Autodesk Inventor part; units mm, degrees
ref_plane "YZ Plane" through (0, 0, 0) normal (1, 0, 0) x (0, 1, 0)
ref_plane "XZ Plane" through (0, 0, 0) normal (0, 1, 0) x (-1, 0, 0)
ref_plane "XY Plane" through (0, 0, 0) normal (0, 0, 1) x (1, 0, 0)
sketch "Szkic3" plane through (0, 0, 0) normal (0, 1, 0) x (-1, 0, 0)
  line L0 (0, 0) -> (10, 0)
  line L1 (10, 0) -> (10, -50)
  line L2 (10, -50) -> (0, -50)
  line L3 (0, -50) -> (0, 0)
  circle A0 centre (5, -5) radius 2.5
  arc A1 (10, -2.5) -> (0, -2.5) centre (5, -6.25) ccw
  line L4 (8, -50) -> (2, -50)
  line L5 (2, -50) -> (2, -10)
  line L6 (2, -10) -> (8, -10)
  line L7 (8, -10) -> (8, -50)
  line L8 (2, -10) -> (8, -16)
  line L9 (2, -10) -> (10.4853, -10) construction
  line L10 (8, -16) -> (8, -18)
  line L11 (8, -18) -> (2, -12)
  line L12 (2, -10) -> (2, -12)
  line L13 (8, -18) -> (8, -22)
  line L14 (2, -16) -> (8, -22)
  line L15 (8, -24) -> (2, -18)
  line L16 (8, -16) -> (8, -14)
  line L17 (8, -24) -> (8, -26)
  line L18 (2, -20) -> (8, -26)
  line L19 (8, -28) -> (2, -22)
  line L20 (8, -28) -> (8, -32)
  line L21 (2, -26) -> (8, -32)
  line L22 (8, -34) -> (2, -28)
  line L23 (8, -34) -> (8, -36)
  line L24 (2, -26) -> (8, -32)
  line L25 (8, -34) -> (2, -28)
  line L26 (8, -34) -> (8, -38)
  line L27 (2, -32) -> (8, -38)
  line L28 (8, -40) -> (2, -34)
  line L29 (8, -40) -> (8, -42)
  line L30 (2, -32) -> (8, -38)
  line L31 (8, -40) -> (2, -34)
  line L32 (8, -40) -> (8, -44)
  line L33 (2, -38) -> (8, -44)
  line L34 (8, -46) -> (2, -40)
  line L35 (8, -46) -> (8, -48)
  line L36 (2, -38) -> (8, -44)
  line L37 (8, -46) -> (2, -40)
  line L38 (8, -46) -> (8, -50)
  line L39 (8, -46) -> (8, -48)
  line L40 (8, -48) -> (2, -42)
  line L41 (2, -42) -> (2, -44)
  line L42 (2, -44) -> (8, -50)
  line L43 (7, -49) -> (2, -49)
  circle A2 centre (5, -5) radius 3.25
  dimension "d9" = 10
  dimension "d10" = 50
  dimension "d11" = 5
  dimension "d12" = 6
  dimension "d13" = 40
  dimension "d14" = 45
  dimension "d15" = 2
  dimension "d16" = 4
  dimension "d17" = 2
  dimension "d18" = 2
  dimension "d19" = 2
  dimension "d20" = 2
  dimension "d21" = 4
  dimension "d22" = 2
  dimension "d23" = 2
  dimension "d24" = 2
  dimension "d25" = 4
  dimension "d26" = 2
  dimension "d27" = 2
  dimension "d28" = 2
  dimension "d29" = 4
  dimension "d30" = 2
  dimension "d32" = 2
  dimension "d36" = 2
  dimension "d37" = 2
  dimension "d42" = 6.5
extrude "Wyciągnięcie proste2" add sketch "Szkic3" against normal blind 2 contours A1 L1 L2 L7 L6 L5 L3 | L5 L43 L42 L2 | L42 L5 L40 L7 | L34 L5 L33 L7 | L28 L5 L27 L7 | L5 L21 L7 L22 | L5 L18 L7 L19 | L5 L14 L7 L15 | L5 L8 L7 L11 | A2
ref_plane "Płaszczyzna konstrukcyjna1" through (0, 0, -50) normal (0, 0, -1) x (-1, 0, 0)
mirror "Odbij1" about plane through (0, 0, -50) normal (0, 0, -1) of "Wyciągnięcie proste2"
sketch "Szkic4" plane through (0, 0, 0) normal (0, 1, 0) x (1, 0, 0)
  line L0 (-7.5, 91.0504) -> (-2.5, 91.0504)
  line L1 (-2.5, 91.0504) -> (-2.5, 98.6571)
  line L2 (-2.5, 98.6571) -> (-7.5, 98.6571)
  line L3 (-7.5, 98.6571) -> (-7.5, 91.0504)
  point P0 (0, 0)
extrude "Wyciągnięcie proste3" cut sketch "Szkic4" against normal blind 2
sketch "Szkic5" plane through (0, 0, 0) normal (0, 1, 0) x (1, 0, 0)
  line L0 (-10, 2.5) -> (-10, 97.5)
  line L1 (-10, 97.5) -> (-10, 67.5)
  line L2 (-10, 67.5) -> (-13, 67.5)
  line L3 (-13, 67.5) -> (-13, 97.5)
  line L4 (-13, 97.5) -> (-10, 97.5)
  arc A0 (0, 97.5) -> (-10, 97.5) centre (-5, 93.75) ccw
  line L5 (-5, 100) -> (-5, 49.8742)
  line L6 (-5, 100) -> (45.1258, 100) construction
  line L7 (-13, 67.5) -> (-10, 62.3038)
  line L8 (-13, 67.5) -> (-7, 67.5) construction
  line L9 (-10, 62.3038) -> (-10, 67.5)
  line L10 (0, 2.5) -> (0, 97.5)
  line L11 (0, 67.5) -> (3, 67.5)
  line L12 (3, 67.5) -> (3, 97.5)
  line L13 (3, 97.5) -> (0, 97.5)
  line L14 (3, 67.5) -> (0, 62.3038)
  arc A1 (3, 97.5) -> (-13, 97.5) centre (-5, 94.4495) ccw
  point P0 (0, 0)
  dimension "d43" = 30
  dimension "d44" = 3
  dimension "d45" = 90
  dimension "d46" = 60
extrude "Wyciągnięcie proste4" add sketch "Szkic5" against normal blind 2
sketch "Szkic6" plane through (0, 0, 0) normal (0, 1, 0) x (1, 0, 0)
  line L0 (-10, 62.3038) -> (-10, 2.5)
  line L1 (-10, 62.3038) -> (-10, 97.356)
  line L2 (-10, 97.356) -> (0, 97.356)
  line L3 (0, 97.356) -> (0, 62.3038)
  line L4 (0, 62.3038) -> (-10, 62.3038)
  point P0 (0, 0)
extrude "Wyciągnięcie proste5" cut sketch "Szkic6" against normal blind 2
sketch "Szkic7" plane through (0, 0, 0) normal (0, 1, 0) x (1, 0, 0)
  line L0 (-10, 62.3038) -> (-8, 62.3038)
  line L1 (-10, 62.3038) -> (-10, 67.4287)
  line L2 (-10, 62.3038) -> (-10, 97.356)
  line L3 (-10, 67.4287) -> (0, 67.4287)
  line L4 (0, 62.3038) -> (0, 97.356)
  line L5 (0, 62.3038) -> (0, 67.4287)
  line L6 (0, 62.3038) -> (-2, 62.3038)
  line L7 (-10, 2.5) -> (-10, 62.3038)
  line L8 (0, 62.3038) -> (-10, 62.3038)
  line L9 (-10, 62.3038) -> (-10, 61.2351)
  line L10 (-10, 61.2351) -> (0, 61.2351)
  line L11 (0, 61.2351) -> (0, 62.3038)
  line L12 (-10, 61.2351) -> (0, 61.2351)
  line L13 (0, 2.5) -> (0, 62.3038)
  line L14 (0, 61.2351) -> (0, 67.4287)
  line L15 (0, 67.4287) -> (-10, 67.4287)
  line L16 (-10, 61.2351) -> (-10, 67.4287)
  point P0 (0, 0)
extrude "Wyciągnięcie proste6" add sketch "Szkic7" against normal blind 2
sketch "Szkic8" plane through (0, 0, 0) normal (0, 1, 0) x (1, 0, 0)
  line L0 (-7.5, 97.356) -> (-10, 97.356)
  line L1 (-10, 97.356) -> (-11, 97.356)
  line L2 (-11, 97.356) -> (-11, 67.4287)
  line L3 (-11, 67.4287) -> (-10, 67.4287)
  line L4 (-10, 67.4287) -> (-10, 97.356)
  line L5 (0, 97.356) -> (1, 97.356)
  line L6 (1, 97.356) -> (1, 67.4287)
  line L7 (1, 67.4287) -> (0, 67.4287)
  line L8 (0, 67.4287) -> (0, 97.356)
  line L9 (-11, 67.4287) -> (1, 67.4287)
  line L10 (1, 67.4287) -> (1, 72.7222)
  line L11 (1, 72.7222) -> (-11, 72.7222)
  line L12 (-11, 72.7222) -> (-11, 67.4287)
  point P0 (0, 0)
  point P1 (0, 72.7222)
  point P2 (-10, 72.7222)
  dimension "d53" = 1
  dimension "d54" = 1
extrude "Wyciągnięcie proste7" cut sketch "Szkic8" against normal blind 2 contours L4 L11 L2 L1 | L8 L5 L6 L11
sketch "Szkic9" plane through (0, 0, 0) normal (0, 1, 0) x (1, 0, 0)
  line L0 (-10, 72.7222) -> (0, 72.7222)
  line L1 (0, 72.7222) -> (0, 67.3617)
  line L2 (0, 67.3617) -> (-10, 67.3617)
  line L3 (-10, 67.3617) -> (-10, 72.7222)
  point P0 (0, 0)
extrude "Wyciągnięcie proste8" add sketch "Szkic9" against normal blind 2
sketch "Szkic10" plane through (0, 0, 0) normal (0, 1, 0) x (1, 0, 0)
  point P0 (0, 0)
split "Podział1" plane through (0, 0, -50) removes the side toward (0, 0, -1)
sketch "Szkic11" plane through (0, 0, 0) normal (0, 1, 0) x (1, 0, 0)
  line L0 (-10, 2.5) -> (-10, 50)
  line L1 (-10, 50) -> (0, 50)
  line L2 (0, 50) -> (0, 100)
  line L3 (0, 100) -> (-10, 100)
  line L4 (-10, 100) -> (-10, 50)
  line L5 (-10, 100) -> (0, 100)
  line L6 (0, 100) -> (0, 124.634)
  line L7 (0, 124.634) -> (-10, 124.634)
  line L8 (-10, 124.634) -> (-10, 100)
  line L9 (-10, 124.634) -> (-11, 124.634)
  line L10 (-11, 124.634) -> (-11, 100)
  line L11 (-11, 100) -> (-10, 100)
  line L12 (-10, 100) -> (-10, 124.634)
  line L13 (0, 124.634) -> (1, 124.634)
  line L14 (1, 124.634) -> (1, 100)
  line L15 (1, 100) -> (0, 100)
  line L16 (0, 100) -> (0, 124.634)
  line L17 (-11, 100) -> (-9, 100) construction
  line L18 (1, 100) -> (3, 100) construction
  line L19 (-11, 124.634) -> (1, 124.634)
  line L20 (1, 124.634) -> (1, 126.634)
  line L21 (1, 126.634) -> (-11, 126.634)
  line L22 (-11, 126.634) -> (-11, 124.634)
  line L23 (-11, 100) -> (-12, 100)
  line L24 (-12, 100) -> (-12, 126.634)
  line L25 (-12, 126.634) -> (-11, 126.634)
  line L26 (-11, 126.634) -> (-11, 100)
  line L27 (1, 126.634) -> (2, 126.634)
  line L28 (2, 126.634) -> (2, 100)
  line L29 (2, 100) -> (1, 100)
  line L30 (1, 100) -> (1, 126.634)
  line L31 (-12, 100) -> (-10, 96.5359)
  line L32 (-12, 100) -> (-8, 100) construction
  line L33 (2, 100) -> (0, 96.5359)
  line L34 (2, 100) -> (6, 100) construction
  point P0 (0, 0)
  dimension "d59" = 10
  dimension "d60" = 50
  dimension "d61" = 10
  dimension "d62" = 24.634
  dimension "d63" = 1
  dimension "d64" = 1
  dimension "d67" = 2
  dimension "d68" = 1
  dimension "d69" = 1
  dimension "d70" = 60
  dimension "d71" = 120
extrude "Wyciągnięcie proste9" add sketch "Szkic11" against normal blind 2 contours L4 L3 L2 L1 | L31 L23 L11 L4 | L2 L15 L29 L33 | L24 L25 L22 L10 L23 | L29 L14 L20 L27 L28 | L9 L22 L21 L20 L13 L7
sketch "Szkic12" plane through (0, 0, 0) normal (0, 1, 0) x (1, 0, 0)
  line L0 (-8, 51.0298) -> (-2, 51.0298)
  line L1 (-2, 51.0298) -> (-2, 96.6875)
  line L2 (-2, 96.6875) -> (-8, 96.6875)
  line L3 (-8, 96.6875) -> (-8, 51.0298)
  line L4 (-8, 51.0298) -> (-2, 54.4939)
  line L5 (-8, 51.0298) -> (-1.0718, 51.0298) construction
  line L6 (-2, 54.4939) -> (-2, 59.4939)
  line L7 (-2, 59.4939) -> (-8, 56.0298)
  line L8 (-8, 51.0298) -> (-8, 56.0298)
  line L9 (-8, 56.0298) -> (-8, 61.0298)
  line L10 (-8, 61.0298) -> (-2, 64.4939)
  line L11 (-2, 64.4939) -> (-2, 69.4939)
  line L12 (-2, 69.4939) -> (-8, 66.0298)
  line L13 (-8, 61.0298) -> (-8, 66.0298)
  line L14 (-8, 66.0298) -> (-2, 69.4939)
  line L15 (-2, 74.4939) -> (-8, 71.0298)
  line L16 (-8, 76.0298) -> (-2, 79.4939)
  line L17 (-2, 84.4939) -> (-8, 81.0298)
  line L18 (-8, 71.0298) -> (-2, 74.4939)
  line L19 (-2, 79.4939) -> (-8, 76.0298)
  line L20 (-8, 81.0298) -> (-2, 84.4939)
  line L21 (-2, 89.4939) -> (-8, 86.0298)
  line L22 (-8, 76.0298) -> (-2, 79.4939)
  line L23 (-2, 84.4939) -> (-8, 81.0298)
  line L24 (-8, 86.0298) -> (-2, 89.4939)
  line L25 (-2, 94.4939) -> (-8, 91.0298)
  point P0 (0, 0)
  dimension "d74" = 30
  dimension "d75" = 5
  dimension "d76" = 5
  dimension "d77" = 5
  dimension "d78" = 5
  dimension "d79" = 5
  dimension "d80" = 5
  dimension "d81" = 5
  dimension "d82" = 5
  dimension "d83" = 5
  dimension "d84" = 5
  dimension "d85" = 5
  dimension "d86" = 5
extrude "Wyciągnięcie proste10" cut sketch "Szkic12" against normal blind 2 contours L3 L7 L1 L4 | L3 L12 L1 L10 | L3 L16 L1 L15 | L3 L21 L1 L17 | L3 L2 L1 L25
properties part number "arm_v1(bez_dokladnych_otworow_montazowych)"
CAD build for the part. Positions are in the model's coordinates, mm. Round coordinates to 2 decimals unless told otherwise and drop trailing zeros. Loops run counter-clockwise (first coordinate to the right, second up) from the corner with the lowest first, then second, coordinate; pieces in that order, holes last. Notation, with made-up numbers: (-35.5, 10) - (-11.5, 10) arc R11 cw to (-11.5, 22) - close; hole circle Ø3 at (10, 53). An arc over 180 degrees is marked (long way). Return JSON: item names as keys, results as strings. Group by question number.
Q1. Band-saw the part on A-A on z = -119. Give the cut face in (x, y).
Q2. Flat gauge pins, fed straight in: pin 1 Ø1 at (y, z) = (-1.5, -95.5) entering from -X; pin 2 Ø0.6 at (y, z) = (-0.5, -42.5) entering from +X; pin 3 Ø0.6 at (x, y) = (-3.5, -1.5) entering from +Z. Where does each tip first touch, or does it go through?
Q3. Drill centre lines: line 1 along X through (y, z) = (-0.9, -56); line 2 along X through (y, z) = (-0.35, -111); line 3 along X through (y, z) = (-1.85, -80). Where is each one in solid material? Low to high. Write a range as [from, to].
Q4. Two-plate mould, pull along Z, no slides. Class faces 1 (the face through (-5, -1, -37)), 2 (the face through (-11.014, -0.986, -98.292)): +Z half, -Z half, draft (parallel to the pull), parting line (faces both ways), or undercut.
Q5. Band-saw the part on C-C on y = -1. Give the number of separate pieces and of enclosed holes in the cut face, plus the area to 3 significant figures.
Q6. Band-saw the part on B-B on z = -5. Give the cut face in (x, y).
Solutions:
{
 "1": {"outline": "(-12, -2) - (-11, -2) - (-11, 0) - (-12, 0) - close; (1, -2) - (2, -2) - (2, 0) - (1, 0) - close"},
 "2": {"pin 1": "stops at x = -10", "pin 2": "stops at x = 0", "pin 3": "stops at z = -0.12"},
 "3": {"line 1": "x = [-10, -8], [-2, 0]", "line 2": "x = [-12, -11], [1, 2]", "line 3": "x = [-10, 0]"},
 "4": {"face 1": "undercut", "face 2": "+Z half"},
 "5": {"separate pieces": "1", "enclosed holes": "15", "area": "763 mm^2"},
 "6": {"outline": "(-10, -2) - (-7.5, -2) - (-7.5, 0) - (-10, 0) - close; (-2.5, -2) - (0, -2) - (0, 0) - (-2.5, 0) - close"}
}
